Input: part model. Units: mm. Frame: model coordinates. Face numbers are marked on the shaded views. Coordinates: 2 decimals unless noted, no trailing zeros. Loops run counter-clockwise (first coordinate to the right, second up) from the corner with the lowest first, then second, coordinate; pieces in that order, holes last.
(1) Line query: L1, parallel to X at y = 548, z = 556.5; L2, parallel to Y at x = 406.5, z = 507; L3, parallel to Z at x = 604, y = 167. Output: solid intervals per line, ascending.
(2) Section C-C, the plane y = 649. Return loops of the section in (x, z), then the cut area to 3 significant figures.
(3) Section B-B, the plane x = 1071.5. Return loops of the section in (y, z), then the cut area to 3 significant figures.
(4) Section D-D, the plane z = 621. Give the number of separate pieces and of enclosed holes in the cut face, then the cut area to 3 significant figures.
(5) Contact query for flat-ended pins moving along their axis: P1, Ø15.5, axis at y = 12, z = 661.5, coming from the -X side; P2, Ø1.5, axis at x = 324, y = 121, coming from the +Z side. Output: stop coordinate, or through.
(6) Section A-A, the plane x = 538. Return loops of the section in (y, z).
(7) Mould query, pull axis Y, two halves, no side actions, for the marked faces 1, 2, 3 and 4. Classes: released by +Y, released by -Y, zero draft, split by the parting line, or undercut.
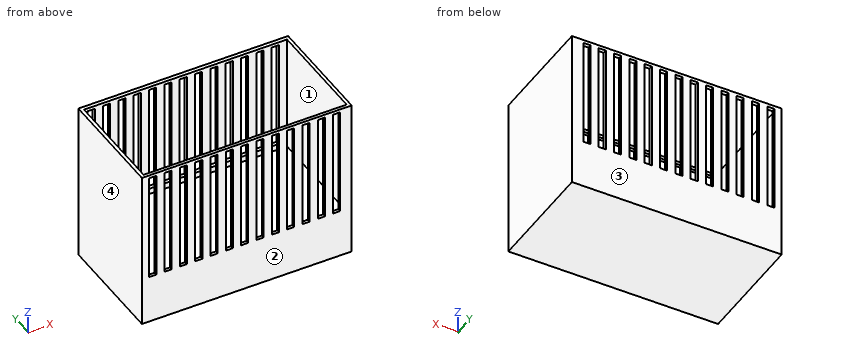
```python
from build123d import *

# Parameters (mm, degrees)
F0_W     = 1300
F0_H     = 700
F1_DEPTH = 1000
F2_W     = 1258.1877
F2_H     = 656.777838
F3_DEPTH = 732.07246
F4_W     = 44.141058
F4_H     = 676.829636
F5_DEPTH = 781.75431


with BuildPart() as f1:
    # F0 (on Top) → F1 (new body)
    with BuildSketch(Plane.XY):
        with Locations((650, 350)):
            Rectangle(F0_W, F0_H)
    extrude(amount=F1_DEPTH)

    # F2 (on face) → F3 (cut)
    with BuildSketch(Plane.XY.offset(1000)):
        with Locations((650.875485, 348.001252)):
            Rectangle(F2_W, F2_H)
    extrude(amount=-F3_DEPTH, mode=Mode.SUBTRACT)

    # F4 (on face) → F5 (cut)
    with BuildSketch(Plane.XZ):
        with Locations((67.042565, 642.217189)):
            Rectangle(F4_W, F4_H)
        with Locations((162.042565, 642.217189)):
            Rectangle(F4_W, F4_H)
        with Locations((257.042565, 642.217189)):
            Rectangle(F4_W, F4_H)
        with Locations((352.042565, 642.217189)):
            Rectangle(F4_W, F4_H)
        with Locations((447.042565, 642.217189)):
            Rectangle(F4_W, F4_H)
        with Locations((542.042565, 642.217189)):
            Rectangle(F4_W, F4_H)
        with Locations((637.042565, 642.217189)):
            Rectangle(F4_W, F4_H)
        with Locations((732.042565, 642.217189)):
            Rectangle(F4_W, F4_H)
        with Locations((827.042565, 642.217189)):
            Rectangle(F4_W, F4_H)
        with Locations((922.042565, 642.217189)):
            Rectangle(F4_W, F4_H)
        with Locations((1017.042565, 642.217189)):
            Rectangle(F4_W, F4_H)
        with Locations((1112.042565, 642.217189)):
            Rectangle(F4_W, F4_H)
        with Locations((1207.042565, 642.217189)):
            Rectangle(F4_W, F4_H)
    extrude(amount=-F5_DEPTH, mode=Mode.SUBTRACT)


solid = f1.part
```
Report:
1. L1: x = 0 to 21.78, 1279.97 to 1300
1. L2: y = 0 to 19.61, 676.39 to 700
1. L3: z = 0 to 267.93
2. outline: (0, 0) - (1300, 0) - (1300, 1000) - (1279.97, 1000) - (1279.97, 267.93) - (21.78, 267.93) - (21.78, 1000) - (0, 1000) - close
2. area: 379,000 mm2
3. outline: (0, 0) - (700, 0) - (700, 1000) - (676.39, 1000) - (676.39, 267.93) - (19.61, 267.93) - (19.61, 1000) - (0, 1000) - close
3. area: 219,000 mm2
4. separate pieces: 26
4. enclosed holes: 0
4. area: 58,800 mm2
5. P1: stops at x = 0
5. P2: stops at z = 267.93
6. outline: (0, 0) - (700, 0) - (700, 303.8) - (676.39, 303.8) - (676.39, 267.93) - (19.61, 267.93) - (19.61, 303.8) - (0, 303.8) - close; (0, 980.63) - (19.61, 980.63) - (19.61, 1000) - (0, 1000) - close; (676.39, 980.63) - (700, 980.63) - (700, 1000) - (676.39, 1000) - close
7. face 1: undercut
7. face 2: released by -Y
7. face 3: released by +Y
7. face 4: zero draft
